Read the model definition and answer for the solid it produces. Units are mm, in the model's axes. Coordinates: 2 decimals unless noted, no trailing zeros. Write each loop counter-clockwise with the first axis right and the second up, starting at its lowest first coordinate (ties: lowest second). Pieces come first, ordered by that corner, then holes. Notation, with made-up numbers: M 25,46 L 55,46 A30 cw 55,80 Z; hole C 23,-10.75 d5. An arc over 180 degrees is marked long. Use a Markdown table: item, result. Add a question column.
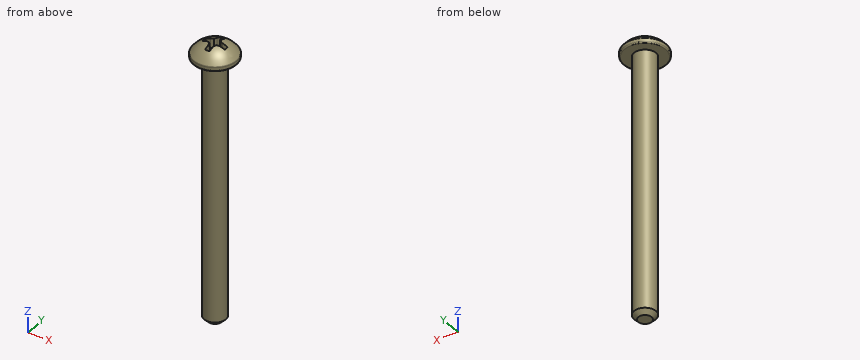
from build123d import *

# Parameters (mm, degrees)
CUT_EXTRUDE1_DEPTH = 1.3563599999999998
DRAFT1_ANGLE       = 15.000000000000034
DRAFT2_ANGLE       = 5.000000000000011


with BuildPart() as part:
    # Sketch2 → Revolve1 (revolve)
    with BuildSketch(Plane(origin=(0, 0, 0), x_dir=(0, 0, -1), z_dir=(1, 0, 0)), mode=Mode.PRIVATE) as revolve1_sk:
        with BuildLine():
            Line((20.1803, -1.04e-15), (20.1803, 0.9525000000000102))
            Line((20.1803, 0.9525000000000102), (19.5453, 1.5875000000000012))
            Line((19.5453, 1.5875000000000012), (-17.919699999999995, 1.5874999999999961))
            Line((-17.919699999999995, 1.5874999999999961), (-17.919699999999995, 2.9500285714285748))
            ThreePointArc((-17.919699999999995, 2.9500285714285748), (-17.96699388646069, 3.064206113539311), (-18.081171428571423, 3.1115000000000004))
            Line((-18.081171428571423, 3.1115000000000004), (-18.513836667869654, 3.1115000000000004))
            ThreePointArc((-18.513836667869654, 3.1115000000000004), (-18.56365651443409, 3.103622207798032), (-18.60861518645835, 3.0807575072424545))
            ThreePointArc((-18.60861518645835, 3.0807575072424545), (-19.76468125738231, 1.7292527267253457), (-20.1803, -1.04e-15))
            Line((-20.1803, -1.04e-15), (20.1803, -1.04e-15))
        make_face()
    revolve(revolve1_sk.sketch.rotate(Axis((0, -1.04e-15, 20.1803), (0, 0, -1)), 90), axis=Axis((0, -1.04e-15, 20.1803), (0, 0, -1)))

    # Sketch3 → Cut-Extrude1 (cut)
    with BuildSketch(Plane.XY.offset(20.1803)):
        with BuildLine():
            Line((0.34999999999999976, 0.8750000000000079), (0.503768939877063, 0.5037689398770607))
            Line((0.503768939877063, 0.5037689398770607), (0.8750000000000099, 0.34999999999999704))
            Line((0.8750000000000099, 0.34999999999999704), (1.7146428199482453, 0.34999999999999704))
            ThreePointArc((1.7146428199482453, 0.34999999999999704), (1.7500000000000198, 3e-17), (1.7146428199482453, -0.34999999999999704))
            Line((1.7146428199482453, -0.34999999999999704), (0.8750000000000099, -0.34999999999999704))
            Line((0.8750000000000099, -0.34999999999999704), (0.503768939877063, -0.5037689398770607))
            Line((0.503768939877063, -0.5037689398770607), (0.34999999999999976, -0.8750000000000079))
            Line((0.34999999999999976, -0.8750000000000079), (0.3499999999999997, -1.7146428199482433))
            ThreePointArc((0.3499999999999997, -1.7146428199482433), (1.1e-16, -1.7500000000000182), (-0.3499999999999997, -1.7146428199482433))
            Line((-0.3499999999999997, -1.7146428199482433), (-0.34999999999999976, -0.8750000000000079))
            Line((-0.34999999999999976, -0.8750000000000079), (-0.503768939877063, -0.5037689398770607))
            Line((-0.503768939877063, -0.5037689398770607), (-0.8750000000000099, -0.34999999999999704))
            Line((-0.8750000000000099, -0.34999999999999704), (-1.7146428199482453, -0.34999999999999704))
            ThreePointArc((-1.7146428199482453, -0.34999999999999704), (-1.7500000000000198, 7.7e-16), (-1.7146428199482453, 0.34999999999999704))
            Line((-1.7146428199482453, 0.34999999999999704), (-0.8750000000000099, 0.34999999999999704))
            Line((-0.8750000000000099, 0.34999999999999704), (-0.503768939877063, 0.5037689398770607))
            Line((-0.503768939877063, 0.5037689398770607), (-0.34999999999999976, 0.8750000000000079))
            Line((-0.34999999999999976, 0.8750000000000079), (-0.3499999999999997, 1.7146428199482433))
            ThreePointArc((-0.3499999999999997, 1.7146428199482433), (1.1e-16, 1.7500000000000182), (0.3499999999999997, 1.7146428199482433))
            Line((0.3499999999999997, 1.7146428199482433), (0.34999999999999976, 0.8750000000000079))
        make_face()
    extrude(amount=-CUT_EXTRUDE1_DEPTH, mode=Mode.SUBTRACT)

    # Draft1
    draft1_faces = [part.faces().sort_by_distance(p)[0] for p in [
        (1.75000000000002, -1.2e-16, 19.288978259234973),
        (1.1e-16, 1.7500000000000182, 19.288978259234973),
        (-1.1e-16, -1.7500000000000182, 19.288978259234973),
        (-1.75000000000002, 1.2e-16, 19.288978259234977),
    ]]
    draft(draft1_faces, Plane.XY.offset(20.1803), DRAFT1_ANGLE)

    # Draft2
    draft2_faces = [part.faces().sort_by_distance(p)[0] for p in [
        (0.34999999999999976, 1.1737349239582926, 19.433218643964523),
        (1.1737349239582928, -0.34999999999999704, 19.43321864396452),
        (0.34999999999999976, -1.1737349239582895, 19.43321864396451),
        (-0.34999999999999976, -1.1737349239582928, 19.433218643964523),
        (-1.1737349236052264, -0.34999999999999704, 19.43321864208228),
        (-1.1737349239582944, 0.34999999999999704, 19.433218643964523),
        (-0.34999999999999976, 1.173734923958288, 19.4332186439645),
        (1.1737349228565852, 0.34999999999999704, 19.433218638091198),
        (0.6881338316552983, 0.4274025012770691, 19.457589851504),
        (0.4274025012770716, 0.6881338316552962, 19.457589851504007),
        (0.6881338316552983, -0.42740250127706914, 19.457589851504004),
        (0.4274025012770716, -0.6881338316552963, 19.457589851504),
        (-0.4274025012770716, -0.6881338316552962, 19.457589851504007),
        (-0.6881338316552983, -0.42740250127706914, 19.457589851504),
        (-0.6881338316552983, 0.4274025012770691, 19.457589851504004),
        (-0.4274025012770716, 0.6881338316552962, 19.457589851504),
    ]]
    draft(draft2_faces, Plane.XY.offset(20.1803), DRAFT2_ANGLE)


solid = part.part
Item 1: Each of these flat-tipped pins is pushed along its axis until it touches: pin 1 (2 mm diameter, centred on x = -2, y = 2.5, fed in from -Z); pin 2 (1.5 mm diameter, centred on x = 2, z = -16, fed in from +Y); pin 3 (1.5 mm diameter, centred on x = 0, z = 9, fed in from +Y). Where does it stop, or does it pass through?
Item 2: Consider probe 1 along Y at (x, z) = (0, 9.5); probe 2 along Y at (x, z) = (-1, 11). Determine where each line is inside the solid, lowest interval first.
Item 3: Find section A-A on z = -17. Give the vertices of the cut face in (x, y) (1 decimal).
Geometry says:
| question | item | result |
|---|---|---|
| 1 | pin 1 | stops at z = 17.92 |
| 1 | pin 2 | stops at y = 0.98 |
| 1 | pin 3 | stops at y = 1.59 |
| 2 | probe 1 | y = -1.59 to 1.59 |
| 2 | probe 2 | y = -1.23 to 1.23 |
| 3 | outline | C 0,0 d3.2 |
